from build123d import *

# Parameters (mm, degrees)
SKETCH_1_W               = 140
SKETCH_1_H               = 80
SKETCH_1_R               = 5
EXTRUDE_1_DEPTH          = 20
EXTRUDE_2_DEPTH          = 80
CUT_EXTRUDE_1_DEPTH      = 65
CUT_EXTRUDE_2_DEPTH      = 41
CUT_EXTRUDE_2_DEPTH_BACK = 41
SKETCH_6_W               = 30
SKETCH_6_H               = 10
CUT_EXTRUDE_3_DEPTH      = 41
CUT_EXTRUDE_3_DEPTH_BACK = 41
SKETCH_7_R               = 25
CUT_EXTRUDE_4_DEPTH      = 35
EXTRUDE_3_DEPTH          = 10
EXTRUDE_3_DEPTH_BACK     = 10


with BuildPart() as part:
    # Эскиз1 → Бобышка-Вытянуть1 (new body)
    with BuildSketch(Plane(origin=(0, 0, 0), x_dir=(1, 0, 0), z_dir=(0, 1, 0))):
        Rectangle(SKETCH_1_W, SKETCH_1_H)
        with Locations((-60, 30)):
            Circle(SKETCH_1_R, mode=Mode.SUBTRACT)
        with Locations((60, 30)):
            Circle(SKETCH_1_R, mode=Mode.SUBTRACT)
        with Locations((60, -30)):
            Circle(SKETCH_1_R, mode=Mode.SUBTRACT)
        with Locations((-60, -30)):
            Circle(SKETCH_1_R, mode=Mode.SUBTRACT)
    extrude(amount=EXTRUDE_1_DEPTH)

    # Эскиз2 → Бобышка-Вытянуть2 (add)
    with BuildSketch(Plane(origin=(0, 20, 0), x_dir=(1, 0, 0), z_dir=(0, 1, 0))):
        with BuildLine():
            Line((-34.003676272, 40), (34.003676272, 40))
            ThreePointArc((34.003676272, 40), (52.5, 0), (34.003676272, -40))
            Line((34.003676272, -40), (-34.003676272, -40))
            ThreePointArc((-34.003676272, -40), (-52.5, 0), (-34.003676272, 40))
        make_face()
    extrude(amount=EXTRUDE_2_DEPTH)

    # Эскиз3 → Вырез-Вытянуть1 (cut)
    with BuildSketch(Plane(origin=(0, 100, 0), x_dir=(1, 0, 0), z_dir=(0, 1, 0))):
        with BuildLine():
            Line((17.5, -21.213203436), (17.5, 21.213203436))
            ThreePointArc((17.5, 21.213203436), (0, 27.5), (-17.5, 21.213203436))
            Line((-17.5, 21.213203436), (-17.5, -21.213203436))
            ThreePointArc((-17.5, -21.213203436), (0, -27.5), (17.5, -21.213203436))
        make_face()
    extrude(amount=-CUT_EXTRUDE_1_DEPTH, mode=Mode.SUBTRACT)

    # Эскиз5 → Вырез-Вытянуть2 (cut, two sides)
    with BuildSketch(Plane.XY) as cut_extrude_2_sk:
        Polygon((-20, 75), (20, 75), (35, 90), (35, 100), (-35, 100), (-35, 90), align=None)
    extrude(amount=CUT_EXTRUDE_2_DEPTH, mode=Mode.SUBTRACT)
    extrude(cut_extrude_2_sk.sketch, amount=-CUT_EXTRUDE_2_DEPTH_BACK, mode=Mode.SUBTRACT)

    # Эскиз6 → Вырез-Вытянуть3 (cut, two sides)
    with BuildSketch(Plane.XY) as cut_extrude_3_sk:
        with Locations((0, 5)):
            Rectangle(SKETCH_6_W, SKETCH_6_H)
    extrude(amount=CUT_EXTRUDE_3_DEPTH, mode=Mode.SUBTRACT)
    extrude(cut_extrude_3_sk.sketch, amount=-CUT_EXTRUDE_3_DEPTH_BACK, mode=Mode.SUBTRACT)

    # Эскиз7 → Вырез-Вытянуть4 (cut)
    with BuildSketch(Plane.XZ):
        Circle(SKETCH_7_R)
    extrude(amount=-CUT_EXTRUDE_4_DEPTH, mode=Mode.SUBTRACT)

    # Эскиз8 → Бобышка-Вытянуть3 (add, two sides)
    with BuildSketch(Plane.XY) as extrude_3_sk:
        Polygon((-70, 20), (-51, 60), (-51, 20), align=None)
        Polygon((51, 60), (51, 20), (70, 20), align=None)
    extrude(amount=EXTRUDE_3_DEPTH)
    extrude(extrude_3_sk.sketch, amount=-EXTRUDE_3_DEPTH_BACK)


solid = part.part
Design review of the part built by this model. Coordinates are the model's own, in mm. A direction names the side the tool comes from. Give positions to 0.01 mm unless a question says otherwise; leave off trailing zeros. Order: outer loops, then holes, each group sorted by start corner. A loop starts at its lowest first (then second) coordinate and runs counter-clockwise, first axis right, second up. Notation, with made-up numbers: (1.25, -0.75) - (53.25, -0.75) arc R27 ccw to (53.25, 15.25) - close; hole circle Ø5 at (46.5, 25). An arc over 180 degrees is marked (long way). Write item = value, one per line. Start each with the question number.
Q1. We need section A-A on x = 0. State the section outline as (y, z) points.
Q2. We need section D-D on x = 59. State the section outline as (y, z) points.
Q3. We need section B-B on z = -8. State the section outline as (x, y) points.
Q4. We need section C-C on y = 32. State the section outline as (x, z) points.
Q5. Clearance check with flat-ended pins moving along their axes: pin 1 Ø1.5 at (y, z) = (31.5, 24.5) entering from -X; pin 2 Ø4 at (y, z) = (69.5, -29.5) entering from -X; pin 3 Ø10.5 at (x, z) = (-4.5, 23.5) entering from +Y; pin 4 Ø6 at (x, z) = (60, -30) entering from -Y. State where each tip first meets the part, or that it passes through.
Q6. To check wall thickness, follow L1, parallel to Z at x = -60, y = 12.75; L2, parallel to X at y = 15.5, z = -30; L3, parallel to X at y = 19, z = 0. State the ranges of each line that lie inside material, in increasing order. Write a range as from..to.
Q7. Mouldability with a two-part tool opening along Z and no side actions: class faces 1 (the face through (-57, 31, 10)), 2 (the face through (0.3, 55.3, -27.5)), 3 (the face through (0, 10, 32)) as released by +Z, released by -Z, zero draft, split by the parting line, or undercut.
Q8. Tool access review of faces 4 (the face through (-18, 75, -1)), 5 (the face through (-52.496, 59.44, 0.637)), 6 (the face through (17.5, 55, 0)), 7 (the face through (56, 20, 25)): name each direction out of +Z, -Z, +X, -X, +Y, -Y from which nothing blocks a thin tool from reaching the whole face with its end or side.
Working result:
q1.outline = (10, -40) - (75, -40) - (75, -27.5) - (35, -27.5) - (35, -25) - (10, -25) - close; (10, 25) - (35, 25) - (35, 27.5) - (75, 27.5) - (75, 40) - (10, 40) - close
q2.outline = (0, -40) - (20, -40) - (20, -34.9) - (0, -34.9) - close; (0, -25.1) - (20, -25.1) - (20, -10) - (43.16, -10) - (43.16, 10) - (20, 10) - (20, 25.1) - (0, 25.1) - close; (0, 34.9) - (20, 34.9) - (20, 40) - (0, 40) - close
q3.outline = (-70, 0) - (-23.69, 0) - (-23.69, 35) - (-17.5, 35) - (-17.5, 75) - (-20, 75) - (-35, 90) - (-35, 100) - (-51.89, 100) - (-51.89, 58.13) - (-70, 20) - close; (17.5, 35) - (23.69, 35) - (23.69, 0) - (70, 0) - (70, 20) - (51.89, 58.13) - (51.89, 100) - (35, 100) - (35, 90) - (20, 75) - (17.5, 75) - close
q4.outline = (-64.3, -10) - (-51.54, -10) arc R52.5 ccw to (-34, -40) - (34, -40) arc R52.5 ccw to (51.54, -10) - (64.3, -10) - (64.3, 10) - (51.54, 10) arc R52.5 ccw to (34, 40) - (-34, 40) arc R52.5 ccw to (-51.54, 10) - (-64.3, 10) - close; hole circle Ø50 at (0, 0)
q5.pin_1 = -46.82
q5.pin_2 = -44.72
q5.pin_3 = 75
q5.pin_4 = through
q6.L1 = -40..-35, -25..25, 35..40
q6.L2 = -70..-65, -55..55, 65..70
q6.L3 = -70..-25, 25..70
q7.face_1 = released by +Z
q7.face_2 = undercut
q7.face_3 = zero draft
q8.face_4 = +Z, -Z, +Y
q8.face_5 = -X, +Y
q8.face_6 = +Y
q8.face_7 = +Z, +X, +Y
